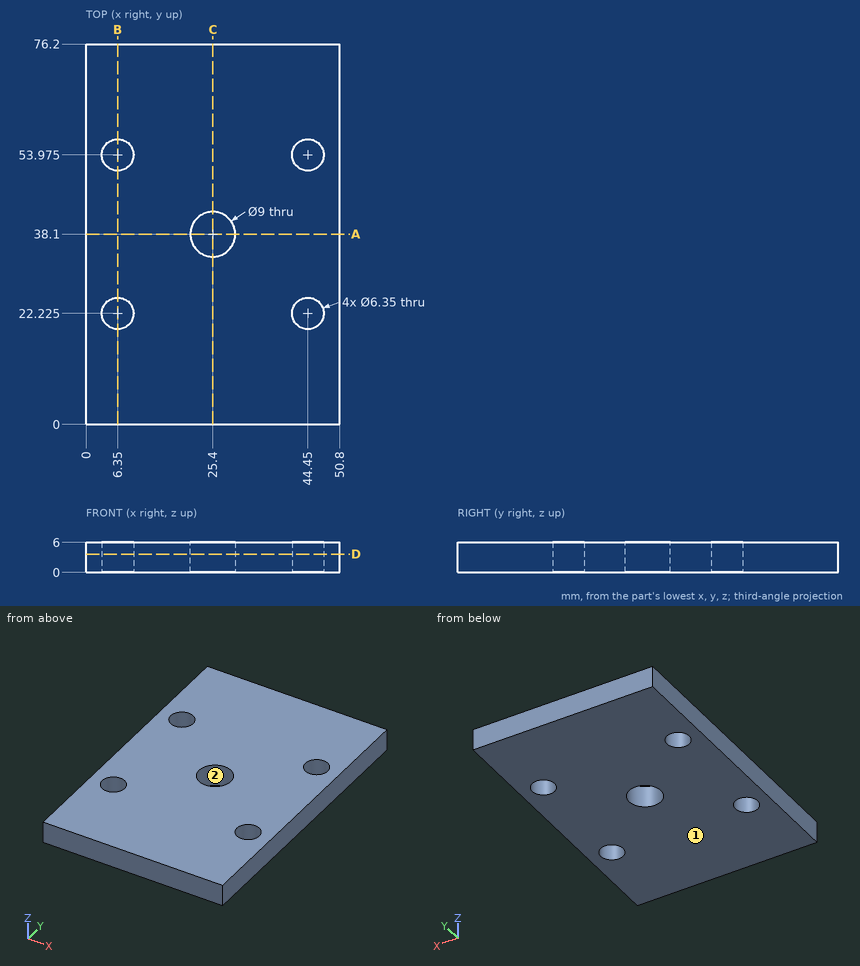
Job drawing, mm, ordinate dimensions from the low corner. One solid piece. Round coordinates to 2 decimals unless told otherwise and drop trailing zeros. Order: outer loops, then holes, each group sorted by start corner. A loop starts at its lowest first (then second) coordinate and runs counter-clockwise, first axis right, second up. Notation, with made-up numbers: M 14,61.25 L 67,61.25 A23 ccw 67,79.25 Z; hole C 72,-34.5 d6. An arc over 180 degrees is marked long. Write each question's results on one line, items separated by ' | '. Start each with the question number.
(1) Saw through at B-B, the plane x = 6.35. Give the cut face in (y, z).
(2) Drop a flat-ended pin along its axis: pin 1 (5 mm diameter, centred on x = 6.35, y = 53.975, fed in from -Z). Give the stop position or say it passes through.
(3) Saw through at C-C, the plane x = 25.4. Give the cut face in (y, z), then the cut area to 3 significant figures.
(4) Probe probe 1 along Y at (x, z) = (44.5, 5.3); probe 2 along Y at (x, z) = (25.4, 4.65); probe 3 along X at (y, z) = (55, 5.3) (3 decimals). List the from-to ranges inside material, lowest first. Write a range as from..to.
(5) Saw through at D-D, the plane z = 3.65. Give the cut face in (x, y) (3 decimals), then the cut area to 3 significant figures.
(6) Saw through at A-A, the plane y = 38.1. Give the cut face in (x, z), then the cut area to 3 significant figures.
(7) Two-plate mould, pull along X, no slides. Class the marked faces 1 and 2: pulls with the +X half, pulls with the -X half, needs draft (parallel to the pull), parting line crosses it, or undercut.
Established:
1) outline: M 0,0 L 19.05,0 L 19.05,6 L 0,6 Z; M 25.4,0 L 50.8,0 L 50.8,6 L 25.4,6 Z; M 57.15,0 L 76.2,0 L 76.2,6 L 57.15,6 Z
2) pin 1: passes through
3) outline: M 0,0 L 33.6,0 L 33.6,6 L 0,6 Z; M 42.6,0 L 76.2,0 L 76.2,6 L 42.6,6 Z | area: 403 mm^2
4) probe 1: y = 0..19.05, 25.4..50.8, 57.15..76.2 | probe 2: y = 0..33.6, 42.6..76.2 | probe 3: x = 0..3.345, 9.355..41.445, 47.455..50.8
5) outline: M 0,0 L 50.8,0 L 50.8,76.2 L 0,76.2 Z; hole C 6.35,22.225 d6.35; hole C 6.35,53.975 d6.35; hole C 25.4,38.1 d9; hole C 44.45,22.225 d6.35; hole C 44.45,53.975 d6.35 | area: 3,680 mm^2
6) outline: M 0,0 L 20.9,0 L 20.9,6 L 0,6 Z; M 29.9,0 L 50.8,0 L 50.8,6 L 29.9,6 Z | area: 251 mm^2
7) face 1: needs draft | face 2: undercut
